Here's how the part is built. I have some questions about the finished solid (model axes, mm). Round coordinates to 2 decimals unless told otherwise and drop trailing zeros. Write each loop counter-clockwise with the first axis right and the second up, starting at its lowest first coordinate (ties: lowest second). Pieces come first, ordered by that corner, then holes. Notation, with made-up numbers: (82, 57) - (139, 57) arc R3 ccw to (139, 62) - close; hole circle Ø6 at (14.25, 52). An arc over 180 degrees is marked (long way). Use one line per item in the form item = value. Start each with the question number.
1. I want a section at B-B, the plane z = 16. List the corners of the cut face in (x, y) for me, plus the area to 3 significant figures.
2. Will this pin go through, and if not, where does the flat tip stop? pin 1 (1 mm diameter, centred on y = 1, z = 12.5, fed in from +X).
3. If I drill on line 1 along Y through (x, z) = (-0.1, 39); line 2 along Z through (x, y) = (-0.05, 4.5); line 3 along Y through (x, z) = (0.4, 39), over which ranges is the centre line in solid material (lowest first)?
4. We'd pull the mould along X, two halves only. Please class faces 1 (the cylindrical face through (0.75, -0.03, 20.34)), 2 (the flat face through (0, 0, 0)): +X half, -X half, draft (parallel to the pull), parting line (faces both ways), or undercut.
5. I want a section at A-A, the plane y = 2.25. List the corners of the cut face in (x, z) for me.
```python
from build123d import *

# Parameters (mm, degrees)
F1_DEPTH     = 42
F2_START     = 40.5
F2_DEPTH     = 1.5
F3_T1_DEPTH  = 8.875
F3_T4_ANGLE  = 180
F3_T8_DEPTH  = 10.75
F3_S9_R      = 0.75
F3_T10_DEPTH = 7
F3_T14_DEPTH = 10.75
F3_S15_R     = 0.75
F3_T16_DEPTH = 7
F4_SIZE2     = 1.299028
F4_SIZE      = 0.74999


# Not quite as in the source:
# - a fillet or chamfer that OpenCascade refuses, or shapes differently, is made with other operations: its cross-section is extruded or revolved along the edge and cut away or added
# - a fillet or chamfer is up to 0.001 mm smaller than in the source, because OpenCascade refuses the exact size


with BuildPart() as f1:
    # F0 (on Top) → F1 (new body)
    with BuildSketch(Plane.XY):
        with BuildLine():
            Line((-0.75, 0), (0.75, 0))
            ThreePointArc((0.75, 0), (0, 0.75), (-0.75, 0))
        make_face()
        with BuildLine():
            ThreePointArc((-0.75, 0), (0, -0.75), (0.75, 0))
            Line((0.75, 0), (-0.75, 0))
        make_face()
    extrude(amount=F1_DEPTH)

    # F0 (on Top) → F2 (join)
    with BuildSketch(Plane.XY.offset(F2_START)):
        with BuildLine():
            ThreePointArc((-0.75, 0), (0, 0.75), (0.75, 0))
            Line((0.75, 0), (0.75, 7))
            Line((0.75, 7), (-0.75, 7))
            Line((-0.75, 7), (-0.75, 0))
        make_face()
    extrude(amount=F2_DEPTH)

    # F3: fillet of radius 0.75 on 5 edges, made by hand

    # F3_s2 → F3_t1 (cut)
    with BuildSketch(Plane.XZ.offset(-8.875)):
        with BuildLine():
            ThreePointArc((0.75, 41.25), (0.5303300859, 41.7803300859), (0, 42))
            Line((0, 42), (0.75, 42))
            Line((0.75, 42), (0.75, 41.25))
        make_face()
        with BuildLine():
            ThreePointArc((0, 42), (-0.5303300859, 41.7803300859), (-0.75, 41.25))
            Line((-0.75, 41.25), (-0.75, 42))
            Line((-0.75, 42), (0, 42))
        make_face()
    extrude(amount=F3_T1_DEPTH, mode=Mode.SUBTRACT)

    # F3_s3 → F3_t4 (revolve, cut)
    with BuildSketch(Plane.XZ):
        with BuildLine():
            ThreePointArc((-0.75, 41.25), (-0.5303300859, 41.7803300859), (0, 42))
            Line((0, 42), (-0.75, 42))
            Line((-0.75, 42), (-0.75, 41.25))
        make_face()
    revolve(axis=Axis((0, 0, 42), (0, 0, 1)), revolution_arc=F3_T4_ANGLE, mode=Mode.SUBTRACT)


with BuildPart() as f3_tool6:
    # F3_s7 → F3_t8 (new body)
    with BuildSketch(Plane.XZ.offset(-8.875)):
        with BuildLine():
            ThreePointArc((0, 40.5), (-0.5303300859, 40.7196699141), (-0.75, 41.25))
            Line((-0.75, 41.25), (-0.75, 40.5))
            Line((-0.75, 40.5), (0, 40.5))
        make_face()
    extrude(amount=F3_T8_DEPTH)

    # F3_s9 → F3_t10 (cut, symmetric)
    with BuildSketch(Plane.XY.offset(40.9)):
        Circle(F3_S9_R)
    extrude(amount=F3_T10_DEPTH, both=True, mode=Mode.SUBTRACT)


with BuildPart() as f1_1:
    add(f1.part)

    # F3_t5: cut F3_tool6
    add(f3_tool6.part, mode=Mode.SUBTRACT)


with BuildPart() as f3_tool12:
    # F3_s13 → F3_t14 (new body)
    with BuildSketch(Plane.XZ.offset(1.875)):
        with BuildLine():
            ThreePointArc((0, 40.5), (0.5303300859, 40.7196699141), (0.75, 41.25))
            Line((0.75, 41.25), (0.75, 40.5))
            Line((0.75, 40.5), (0, 40.5))
        make_face()
    extrude(amount=-F3_T14_DEPTH)

    # F3_s15 → F3_t16 (cut, symmetric)
    with BuildSketch(Plane.XY.offset(40.9)):
        Circle(F3_S15_R)
    extrude(amount=F3_T16_DEPTH, both=True, mode=Mode.SUBTRACT)


with BuildPart() as f1_2:
    add(f1_1.part)

    # F3_t11: cut F3_tool12
    add(f3_tool12.part, mode=Mode.SUBTRACT)

    # F4 (size 0.75 and 1.2990381057 in the source; OpenCascade refuses exactly that, so slightly less here)
    f4_edges = [f1_2.edges().sort_by_distance(p)[0] for p in [
        (-0.53033, 7, 40.71967),
        (0.53033, 7, 40.71967),
        (-0.53033, 7, 41.78033),
        (0.53033, 7, 41.78033),
    ]]
    f4_side = f1_2.faces().sort_by_distance((0, 7, 41.25))[0]
    chamfer(f4_edges, length=F4_SIZE, length2=F4_SIZE2, reference=f4_side)


solid = f1_2.part
```
Model answer:
q1.outline = circle Ø1.5 at (0, 0)
q1.area = 1.77 mm2
q2.pin_1 = 0.56
q3.line_1 = -0.74 to 0.74
q3.line_2 = 40.5 to 42
q3.line_3 = -0.63 to 0.63
q4.face_1 = parting line
q4.face_2 = draft
q5.outline = circle Ø1.5 at (0, 41.25)
